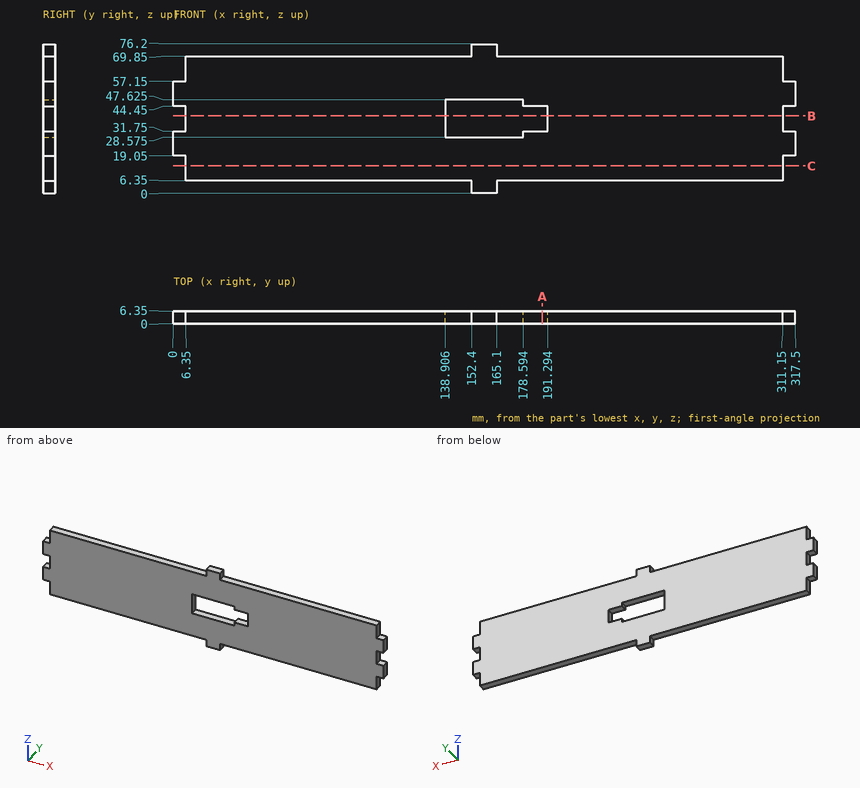
Job drawing, mm, ordinate dimensions from the low corner. One solid piece. Round coordinates to 2 decimals unless told otherwise and drop trailing zeros. Write each loop counter-clockwise with the first axis right and the second up, starting at its lowest first coordinate (ties: lowest second). Pieces come first, ordered by that corner, then holes.
1) Band-saw the part on C-C, the plane z = 14. List the corners of the cut face in (x, y).
2) Band-saw the part on B-B, the plane z = 39.5. List the corners of the cut face in (x, y), and give its area (3 significant figures).
3) Drill centre lines: probe 1 along Z at (x, y) = (163, 5) (1 decimal); probe 2 along X at (y, z) = (5.5, 39.5); probe 3 along Z at (x, y) = (252.5, 5). Where is each one in solid material? Low to high.
4) Band-saw the part on A-A, the plane x = 188.5. List the corners of the cut face in (y, z), and give its area (3 significant figures).
5) Pin check, flat tips, straight feed: pin 1 (1.9 mm diameter, centred on x = 3.5, y = 3.5, fed in from -Z); pin 2 (2 mm diameter, centred on y = 5.5, z = 67.5, fed in from +X); pin 3 (1.9 mm diameter, centred on y = 2, z = 2, fed in from -X). Stop position of each tip, or through.
Ans:
1. outline: (6.35, 0) - (311.15, 0) - (311.15, 6.35) - (6.35, 6.35) - close
2. outline: (6.35, 0) - (138.91, 0) - (138.91, 6.35) - (6.35, 6.35) - close; (191.29, 0) - (311.15, 0) - (311.15, 6.35) - (191.29, 6.35) - close
2. area: 1,600 mm2
3. probe 1: z = 0 to 28.6, 47.6 to 76.2
3. probe 2: x = 6.35 to 138.91, 191.29 to 311.15
3. probe 3: z = 6.35 to 69.85
4. outline: (0, 6.35) - (6.35, 6.35) - (6.35, 31.75) - (0, 31.75) - close; (0, 44.45) - (6.35, 44.45) - (6.35, 69.85) - (0, 69.85) - close
4. area: 323 mm2
5. pin 1: stops at z = 19.05
5. pin 2: stops at x = 311.15
5. pin 3: stops at x = 152.4
